```python
from build123d import *

# Parameters (mm, degrees)
CROQUIS1_R              = 18.4
SALIENTE_EXTRUIR1_DEPTH = 26.3
CROQUIS2_R              = 3
CROQUIS2_R_2            = 1.25
CORTAR_EXTRUIR1_DEPTH   = 5
CROQUIS3_R              = 1.25
CORTAR_EXTRUIR2_DEPTH   = 5
CROQUIS7_R              = 18.4
CORTAR_EXTRUIR5_DEPTH   = 19.3
CROQUIS8_R              = 6
CORTAR_EXTRUIR6_DEPTH   = 1


with BuildPart() as part:
    # Croquis1 → Saliente-Extruir1 (new body)
    with BuildSketch(Plane.XY):
        Circle(CROQUIS1_R)
    extrude(amount=SALIENTE_EXTRUIR1_DEPTH)

    # Croquis2 → Cortar-Extruir1 (cut)
    with BuildSketch(Plane.XY.offset(26.3)):
        Circle(CROQUIS2_R)
        with Locations((0, 9.5)):
            Circle(CROQUIS2_R_2)
        with Locations((9.5, 0)):
            Circle(CROQUIS2_R_2)
        with Locations((0, -9.5)):
            Circle(CROQUIS2_R_2)
        with Locations((-9.5, 0)):
            Circle(CROQUIS2_R_2)
    extrude(amount=-CORTAR_EXTRUIR1_DEPTH, mode=Mode.SUBTRACT)

    # Croquis3 → Cortar-Extruir2 (cut)
    with BuildSketch(Plane(origin=(0, 0, 0), x_dir=(-1, 0, 0), z_dir=(0, 0, -1))):
        with Locations((-10, 0)):
            Circle(CROQUIS3_R)
        with Locations((0, 10)):
            Circle(CROQUIS3_R)
        with Locations((10, 0)):
            Circle(CROQUIS3_R)
        with Locations((0, -10)):
            Circle(CROQUIS3_R)
    extrude(amount=-CORTAR_EXTRUIR2_DEPTH, mode=Mode.SUBTRACT)

    # Croquis7 → Cortar-Extruir5 (cut)
    with BuildSketch(Plane(origin=(0, 0, 0), x_dir=(-1, 0, 0), z_dir=(0, 0, -1))):
        Circle(CROQUIS7_R)
    extrude(amount=-CORTAR_EXTRUIR5_DEPTH, mode=Mode.SUBTRACT)

    # Croquis8 → Cortar-Extruir6 (cut)
    with BuildSketch(Plane(origin=(0, 0, 19.3), x_dir=(-1, 0, 0), z_dir=(0, 0, -1))):
        Circle(CROQUIS8_R)
    extrude(amount=-CORTAR_EXTRUIR6_DEPTH, mode=Mode.SUBTRACT)


solid = part.part
```
Can you work these out from the model? Positions are in its coordinate system, mm. A direction names the side the tool comes from. Round coordinates to 2 decimals unless told otherwise and drop trailing zeros. Order: outer loops, then holes, each group sorted by start corner. A loop starts at its lowest first (then second) coordinate and runs counter-clockwise, first axis right, second up. Notation, with made-up numbers: (16, -6) -> (41, -6) arc R30 cw to (41, 32) -> close; hole circle Ø2 at (37, 14). An arc over 180 degrees is marked (long way). Return JSON: item names as keys, results as strings. Group by question number.
1. If we section it at A-A, the plane z = 23: Write out the boundary of the cut face in (x, y).
2. Will these pins go through, and if not, where does the flat tip stop? pin 1 (0.8 mm diameter, centred on x = 0, y = 9, fed in from +Z); pin 2 (4 mm diameter, centred on y = 8, z = 24.5, fed in from -X); pin 3 (2 mm diameter, centred on y = 11.5, z = 25, fed in from -X); pin 4 (2 mm diameter, centred on x = -14.5, y = 13.5, fed in from -Z).
3. If we section it at B-B, the plane y = 0: Write out the boundary of the cut face in (x, z), then the cut area to 3 significant figures.
4. Which directions (+Z, -Z, +X, -X, +Y, -Y) give clear straight access to the entire face, cutting with the end or side of a thin tool? Please do faces 5 (the face through (-10, 0, 21.3)), 6 (the face through (0, 0, 20.3)), 7 (the face through (0, -4, 26.3)).
5. We'd pull the mould along Y, two halves only. Please class faces 1 (the face through (-14.6, -11.2, 22.8)), 2 (the face through (0, -9, 21.3)), 3 (the face through (4.35, 4.35, 19.3)), 4 (the face through (-3, 0, 24)): released by +Y, released by -Y, zero draft, split by the parting line, or undercut.
6. I need wall thicknesses on line 1 (Y direction, x = -1, z = 22); line 2 (X direction, y = 9, z = 24). Which ranges of each line are inside material? Lowest first, please. Write a range as [from, to].
7. If we section it at C-C, the plane x = -4.5: Write out the boundary of the cut face in (y, z).
Output values:
{
 "1": {"outline": "circle Ø36.8 at (0, 0); hole circle Ø2.5 at (-9.5, 0); hole circle Ø6 at (0, 0); hole circle Ø2.5 at (0, -9.5); hole circle Ø2.5 at (0, 9.5); hole circle Ø2.5 at (9.5, 0)"},
 "2": {"pin 1": "z = 21.3", "pin 2": "x = -17.39", "pin 3": "x = -15.11", "pin 4": "through"},
 "3": {"outline": "(-18.4, 19.3) -> (-6, 19.3) -> (-6, 20.3) -> (6, 20.3) -> (6, 19.3) -> (18.4, 19.3) -> (18.4, 26.3) -> (10.75, 26.3) -> (10.75, 21.3) -> (8.25, 21.3) -> (8.25, 26.3) -> (3, 26.3) -> (3, 21.3) -> (-3, 21.3) -> (-3, 26.3) -> (-8.25, 26.3) -> (-8.25, 21.3) -> (-10.75, 21.3) -> (-10.75, 26.3) -> (-18.4, 26.3) -> close", "area": "191 mm²"},
 "4": {"face 5": "+Z", "face 6": "-Z", "face 7": "+Z, +X, -X, +Y, -Y"},
 "5": {"face 1": "split by the parting line", "face 2": "undercut", "face 3": "zero draft", "face 4": "undercut"},
 "6": {"line 1": "[-18.37, -10.25], [-8.75, -2.83], [2.83, 8.75], [10.25, 18.37]", "line 2": "[-16.05, -1.15], [1.15, 16.05]"},
 "7": {"outline": "(-17.84, 19.3) -> (-3.97, 19.3) -> (-3.97, 20.3) -> (3.97, 20.3) -> (3.97, 19.3) -> (17.84, 19.3) -> (17.84, 26.3) -> (-17.84, 26.3) -> close"}
}
